```python
from build123d import *

# Parameters (mm, degrees)
SKETCH1_R           = 7
SKETCH1_R_2         = 2.5
BOSS_EXTRUDE1_DEPTH = 5
SKETCH2_R           = 6
CUT_EXTRUDE1_DEPTH  = 0.1
SKETCH3_R           = 6
CUT_EXTRUDE2_DEPTH  = 0.1
CHAMFER1_SIZE       = 0.1


with BuildPart() as part:
    # Sketch1 → Boss-Extrude1 (new body)
    with BuildSketch(Plane(origin=(0, 0, 0), x_dir=(1, 0, 0), z_dir=(0, 1, 0))):
        Circle(SKETCH1_R)
        Circle(SKETCH1_R_2, mode=Mode.SUBTRACT)
    extrude(amount=BOSS_EXTRUDE1_DEPTH)

    # Sketch2 → Cut-Extrude1 (cut)
    with BuildSketch(Plane(origin=(0, 5, 0), x_dir=(1, 0, 0), z_dir=(0, 1, 0))):
        Circle(SKETCH2_R)
    extrude(amount=-CUT_EXTRUDE1_DEPTH, mode=Mode.SUBTRACT)

    # Sketch3 → Cut-Extrude2 (cut)
    with BuildSketch(Plane.XZ):
        Circle(SKETCH3_R)
    extrude(amount=-CUT_EXTRUDE2_DEPTH, mode=Mode.SUBTRACT)

    # Chamfer1
    chamfer1_edges = [part.edges().sort_by_distance(p)[0] for p in [
        (-7, 0, 0),
        (-7, 5, 0),
    ]]
    chamfer(chamfer1_edges, length=CHAMFER1_SIZE)


solid = part.part
```
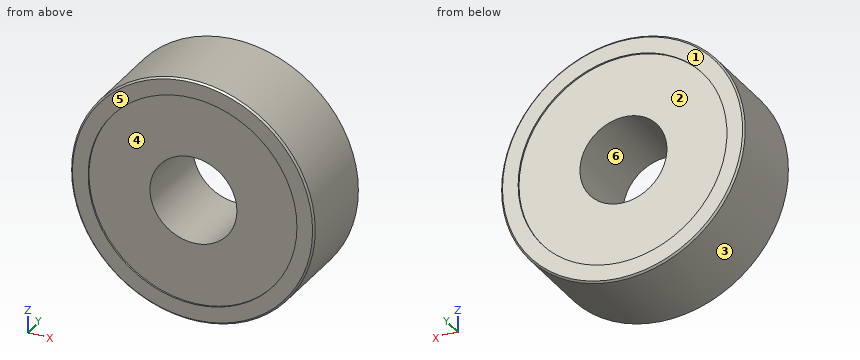
The listing builds one solid part. Answer for the finished solid, in the listing's coordinates (mm). Face numbers are marked on the shaded views. A direction names the side the tool comes from. Coordinates: 2 decimals unless noted, no trailing zeros. Loops run counter-clockwise (first coordinate to the right, second up) from the corner with the lowest first, then second, coordinate; pieces in that order, holes last. Notation, with made-up numbers: (87.25, 47) -> (100.25, 47) arc R22 cw to (100.25, 74) -> close; hole circle Ø2 at (20.5, 85.25). An arc over 180 degrees is marked (long way). Use one line per item in the form item = value. Start each with the question number.
Item 1: The part is cut by section B-B on z = 0. Determine the outline of the cut face in (x, y), then the cut area to 3 significant figures.
Item 2: The mould has two halves that part along Z. Classify the marked faces 3, 4, 5 and 6: released by +Z, released by -Z, zero draft, split by the parting line, or undercut.
Item 3: A tool of negligible diameter and unlimited length cuts with its end or side. For the marked faces 1 and 2, from which of +Z, -Z, +X, -X, +Y, -Y can it reach the whole face along a straight path? Write none if from no direction.
Item 4: The part is cut by section A-A on x = 0. Determine the outline of the cut face in (y, z).
Item 5: The part is cut by section C-C on y = 2.15. Determine the outline of the cut face in (x, z), then the cut area to 3 significant figures.
Item 6: Flat-ended cylindrical pins translate along their axes: pin 1 Ø1.5 at (x, y) = (-4, 4) entering from +Z; pin 2 Ø1.5 at (y, z) = (3, -4.5) entering from -X; pin 3 Ø1 at (x, y) = (-4, 2) entering from -Z; pin 4 Ø4.5 at (x, z) = (0, 0) entering from -Y. Find the tip coordinate at first contact, or state that the pin passes through.
Item 7: Consider L1, parallel to Y at x = -2.5, z = -3.5; L2, parallel to Z at x = -1.5, y = 2.3; L3, parallel to X at y = 1.6, z = 1. Determine where each line is inside the solid, lowest interval first. Write a range as [from, to].
Answer key:
q1.outline = (-7, 0.1) -> (-6.9, 0) -> (-6, 0) -> (-6, 0.1) -> (-2.5, 0.1) -> (-2.5, 4.9) -> (-6, 4.9) -> (-6, 5) -> (-6.9, 5) -> (-7, 4.9) -> close; (2.5, 0.1) -> (6, 0.1) -> (6, 0) -> (6.9, 0) -> (7, 0.1) -> (7, 4.9) -> (6.9, 5) -> (6, 5) -> (6, 4.9) -> (2.5, 4.9) -> close
q1.area = 43.6 mm2
q2.face_3 = split by the parting line
q2.face_4 = undercut
q2.face_5 = zero draft
q2.face_6 = undercut
q3.face_1 = +Z, -Z, +X, -X, +Y
q3.face_2 = +Y
q4.outline = (0, -6.9) -> (0.1, -7) -> (4.9, -7) -> (5, -6.9) -> (5, -6) -> (4.9, -6) -> (4.9, -2.5) -> (0.1, -2.5) -> (0.1, -6) -> (0, -6) -> close; (0, 6) -> (0.1, 6) -> (0.1, 2.5) -> (4.9, 2.5) -> (4.9, 6) -> (5, 6) -> (5, 6.9) -> (4.9, 7) -> (0.1, 7) -> (0, 6.9) -> close
q5.outline = circle Ø14 at (0, 0); hole circle Ø5 at (0, 0)
q5.area = 134 mm2
q6.pin_1 = 6.2
q6.pin_2 = -5.91
q6.pin_3 = -6.06
q6.pin_4 = through
q7.L1 = [0.1, 4.9]
q7.L2 = [-6.84, -2], [2, 6.84]
q7.L3 = [-6.93, -2.29], [2.29, 6.93]
